For this review, take the finished solid that the model builds, in its own axes (mm). Face numbers are marked on the shaded views. A direction names the side the tool comes from. Give positions to 0.01 mm unless a question says otherwise; leave off trailing zeros. Loops run counter-clockwise (first coordinate to the right, second up) from the corner with the lowest first, then second, coordinate; pieces in that order, holes last. Notation, with made-up numbers: (61.25, 48.25) - (72.25, 48.25) arc R23 ccw to (72.25, 61.25) - close; hole circle Ø6 at (-18.75, 74.5). An arc over 180 degrees is marked (long way). Answer in a Markdown table with one row per item.
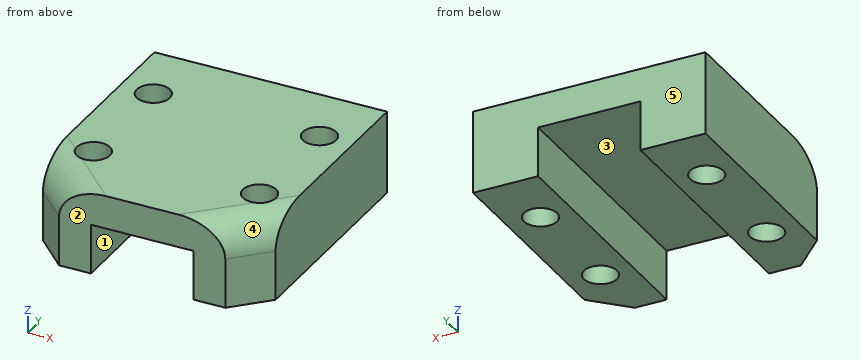
Autodesk Inventor part; units mm, degrees
ref_plane "YZ Plane" through (0, 0, 0) normal (1, 0, 0) x (0, 1, 0)
ref_plane "XZ Plane" through (0, 0, 0) normal (0, 1, 0) x (-1, 0, 0)
ref_plane "XY Plane" through (0, 0, 0) normal (0, 0, 1) x (1, 0, 0)
sketch "Sketch1" plane through (0, 0, 0) normal (0, 0, 1) x (1, 0, 0)
  line L0 (7, 7.5) -> (3, 7.5)
  line L1 (3, 7.5) -> (3, -7.5)
  line L2 (7, -7.5) -> (3, -7.5)
  line L3 (7, 7.5) -> (7, -7.5)
  circle A0 centre (5, -3.5) radius 1
  circle A1 centre (5, 3.5) radius 1
  line L4 (-3, 7.5) -> (-7, 7.5)
  line L5 (-7, -7.5) -> (-7, 7.5)
  line L6 (-3, -7.5) -> (-7, -7.5)
  line L7 (-3, -7.5) -> (-3, 7.5)
  circle A2 centre (-5, 3.5) radius 1
  circle A3 centre (-5, -3.5) radius 1
  point P0 (0, 0)
extrude "Extrusion1" add sketch "Sketch1" along normal blind 3
sketch "Sketch2" plane through (0, 0, 3) normal (0, 0, 1) x (1, 0, 0)
  line L0 (7, -7.5) -> (7, 7.5)
  line L1 (7, 7.5) -> (3, 7.5)
  line L2 (3, 7.5) -> (3, -7.5)
  line L3 (3, -7.5) -> (7, -7.5)
  circle A0 centre (5, -3.5) radius 1
  circle A1 centre (5, 3.5) radius 1
  line L4 (-3, -7.5) -> (-3, 7.5)
  line L5 (-3, 7.5) -> (-7, 7.5)
  line L6 (-7, 7.5) -> (-7, -7.5)
  line L7 (-7, -7.5) -> (-3, -7.5)
  circle A2 centre (-5, 3.5) radius 1
  circle A3 centre (-5, -3.5) radius 1
  line L8 (7, -7.5) -> (-7, -7.5)
  line L9 (-7, -7.5) -> (-7, 7.5)
  line L10 (-7, 7.5) -> (7, 7.5)
  line L11 (7, 7.5) -> (7, -7.5)
  point P0 (0, 0)
extrude "Extrusion2" add sketch "Sketch2" along normal blind 2
chamfer "Chamfer1" distance 2 angle 45 2 edges at (7, -7.5, 2.5) (-7, -7.5, 2.5)
fillet "Fillet1" radius 2 2 edges at (6, -6.5, 5) (-6, -6.5, 5)
thicken "Thicken1" operation add thickness 0.08 both sides no extend neighbours yes toward (-1, 0, 0) faces at (-3, -2.5, 1)
thicken "Thicken2" operation add thickness 0.08 both sides no extend neighbours yes toward (1, 0, 0) faces at (3, 2.5, 1)
properties part number "sub_arm_2_mod"
1. We need section A-A, the plane y = 3.5. Give the boundary of the cut face in (x, z), and give its area (3 significant figures).
Values:
| item | result |
|---|---|
| outline | (-7, 0) - (-6, 0) - (-6, 5) - (-7, 5) - close; (-4, 0) - (-3.08, 0) - (-3.08, 3) - (3.08, 3) - (3.08, 0) - (4, 0) - (4, 5) - (-4, 5) - close; (6, 0) - (7, 0) - (7, 5) - (6, 5) - close |
| area | 31.5 mm^2 |
2. We need section B-B, the plane z = 1.05. Give the boundary of the cut face in (x, y), and give its area (3 significant figures).
Values:
| item | result |
|---|---|
| outline | (-7, -5.5) - (-5, -7.5) - (-3.08, -7.5) - (-3.08, 7.5) - (-7, 7.5) - close; (3.08, -7.5) - (5, -7.5) - (7, -5.5) - (7, 7.5) - (3.08, 7.5) - close; hole circle Ø2 at (-5, -3.5); hole circle Ø2 at (-5, 3.5); hole circle Ø2 at (5, -3.5); hole circle Ø2 at (5, 3.5) |
| area | 101 mm^2 |
3. For the marked faces 1 and 2, list the 3-axis set-ups (+Z, -Z, +X, -X, +Y, -Y) from which the entire face can be reached by the end or side of a thin tool; tool diameter is ignored.
Values:
| item | result |
|---|---|
| face 1 | -Z, +Y, -Y |
| face 2 | +Z, -Z, +X, -X, -Y |
4. Mouldability with a two-part tool opening along X and no side actions: class the marked faces 3, 4 and 5 as released by +X, released by -X, zero draft, split by the parting line, or undercut.
Values:
| item | result |
|---|---|
| face 3 | undercut |
| face 4 | released by +X |
| face 5 | zero draft |
5. We need section D-D, the plane y = -3.5. Count the separate pieces of the cut face and the enclosed holes in it, and give its area (3 significant figures).
Values:
| item | result |
|---|---|
| separate pieces | 3 |
| enclosed holes | 0 |
| area | 31.5 mm^2 |
6. Wall thickness on line 1 (X direction, y = -3.5, z = 2.6); line 2 (X direction, y = -3, z = 4.7); line 3 (Y direction, x = 5, z = 3.4): over which ranges is each line inside the solid? List them lowest first. Write a range as [from, to].
Values:
| item | result |
|---|---|
| line 1 | x = [-7, -6], [-4, -3.08], [3.08, 4], [6, 7] |
| line 2 | x = [-7, -5.87], [-4.13, 4.13], [5.87, 7] |
| line 3 | y = [-7.44, -4.5], [-2.5, 2.5], [4.5, 7.5] |
7. We need section C-C, the plane z = 3.3. Give the boundary of the cut face in (x, y).
Values:
| item | result |
|---|---|
| outline | (-7, -5.47) - (-4.97, -7.5) - (4.97, -7.5) - (7, -5.47) - (7, 7.5) - (-7, 7.5) - close; hole circle Ø2 at (-5, -3.5); hole circle Ø2 at (-5, 3.5); hole circle Ø2 at (5, -3.5); hole circle Ø2 at (5, 3.5) |
